Design review of the part built by this model. Coordinates are the model's own, in mm. Face numbers are marked on the shaded views. Coordinates: 2 decimals unless noted, no trailing zeros. Write each loop counter-clockwise with the first axis right and the second up, starting at its lowest first coordinate (ties: lowest second). Pieces come first, ordered by that corner, then holes.
Q1. Take a section at A-A (z = 2.75). Give the boundary of the cut face in (x, y), and give its area (3 significant figures).
Q2. For probe 1 along Y at (x, z) = (0, 1.2); probe 2 along Y at (x, z) = (13, 7.5); probe 3 along Z at (x, y) = (13, -13), list the stretches that pass through material, from the lowest coordinate up.
Q3. Mouldability with a two-part tool opening along Y and no side actions: class the marked faces 1 and 2 as pulls with the +Y half, pulls with the -Y half, needs draft (parallel to the pull), parting line crosses it, or undercut.
Q4. Insertion check: pin 1 (8 mm diameter, centred on x = -7, z = 11, fed in from -Y); pin 2 (22 mm diameter, centred on x = -8, y = -10, fed in from +Z); pin 3 (1 mm diameter, centred on y = -14, z = 3, fed in from -X). Each pin has a flat end and moves straight along its axis. Give the tip position at first contact, or say it passes through.
```python
from build123d import *

# Parameters (mm, degrees)
F2_R = 1.27
F3_T = -1.5


with BuildPart() as f1:
    # F0 (on Front) → F1 (revolve)
    with BuildSketch(Plane.XZ):
        Polygon((-23.5, 0), (0, 0), (0, 5.9944), (-20.828, 5.9944), (-23.5, 5.9944), align=None)
        Polygon((-20.828, 5.9944), (0, 5.9944), (0, 7.366), (-18.1559962, 7.366), (-20.828, 7.366), align=None)
        with BuildLine():
            Line((-18.1559962, 7.366), (0, 7.366))
            Line((0, 7.366), (0, 13.462))
            ThreePointArc((0, 13.462), (-9.3803005465, 12.2615564285), (-18.1559962, 8.7376))
            Line((-18.1559962, 8.7376), (-18.1559962, 7.366))
        make_face()
    revolve(axis=Axis((0, 0, 6.731), (0, 0, 1)))

    # F2
    f2_edges = [f1.edges().sort_by_distance(p)[0] for p in [
        (20.828, 0, 7.366),
        (18.155996, 0, 8.7376),
        (23.5, 0, 5.9944),
    ]]
    fillet(f2_edges, radius=F2_R)

    # F3
    f3_openings = [f1.faces().sort_by_distance(p)[0] for p in [
        (0, 0, 0),
    ]]
    offset(amount=F3_T, openings=f3_openings, kind=Kind.INTERSECTION)


solid = f1.part
```
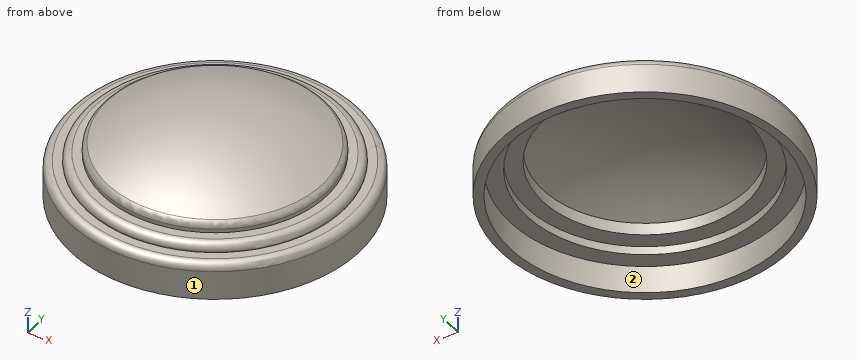
Response:
1. outline: circle Ø47 at (0, 0); hole circle Ø44 at (0, 0)
1. area: 214 mm2
2. probe 1: y = -23.5 to -22, 22 to 23.5
2. probe 2: y = -12.67 to -10.41, 10.41 to 12.67
2. probe 3: z = 5.87 to 7.37
3. face 1: parting line crosses it
3. face 2: undercut
4. pin 1: stops at y = -19.4
4. pin 2: stops at z = 13.42
4. pin 3: stops at x = -19.24
